Could you check a few things on this model? Use its own coordinates, in mm. A direction names the side the tool comes from. Coordinates: 2 decimals unless noted, no trailing zeros. Write each loop counter-clockwise with the first axis right and the second up, starting at its lowest first coordinate (ties: lowest second). Pieces come first, ordered by that corner, then holes.
```python
from build123d import *

# Parameters (mm, degrees)
CROQUIS1_W                = 5
CROQUIS1_H                = 53
SALIENTE_EXTRUIR1_DEPTH   = 7
SALIENTE_EXTRUIR1_2_DEPTH = 7
CROQUIS3_W                = 53
CROQUIS3_H                = 48
CROQUIS3_W_2              = 33
CROQUIS3_H_2              = 33
CROQUIS3_H_3              = 5
SALIENTE_EXTRUIR2_DEPTH   = 5
CROQUIS4_W                = 53
CROQUIS4_H                = 53
CROQUIS4_W_2              = 43
CROQUIS4_H_2              = 43
SALIENTE_EXTRUIR3_DEPTH   = 32
REDONDEO1_R               = 2
REDONDEO2_R               = 5
CROQUIS5_W                = 5
CROQUIS5_H                = 14
CORTAR_EXTRUIR1_DEPTH     = 32
CROQUIS6_W                = 5
CROQUIS6_H                = 6
CORTAR_EXTRUIR2_DEPTH     = 20
REDONDEO3_R               = 2
CROQUIS7_R                = 4
CROQUIS7_R_2              = 1.75
SALIENTE_EXTRUIR4_DEPTH   = 3
REDONDEO4_R               = 3
REDONDEO7_R               = 3


with BuildPart() as part:
    # Croquis1 → Saliente-Extruir1 (new body)
    with BuildSketch(Plane(origin=(0, 0, 0), x_dir=(0, 1, 0), z_dir=(0, 0, 1))):
        with Locations((-24, 0)):
            Rectangle(CROQUIS1_W, CROQUIS1_H)
    extrude(amount=SALIENTE_EXTRUIR1_DEPTH)



with BuildPart() as body_2:
    # Croquis1 → Saliente-Extruir1 2 (new body)
    with BuildSketch(Plane(origin=(0, 0, 0), x_dir=(0, 1, 0), z_dir=(0, 0, 1))):
        with Locations((24, 0)):
            Rectangle(CROQUIS1_W, CROQUIS1_H)
    extrude(amount=SALIENTE_EXTRUIR1_2_DEPTH)


with BuildPart() as part_1:
    add(part.part)

    add(body_2.part)  # Saliente-Extruir2 merges body 2
    # Croquis3 → Saliente-Extruir2 (add)
    # profile 1 of 2: a face of its own
    with BuildSketch(Plane.XY.offset(7)):
        with Locations((0, 2.5)):
            Rectangle(CROQUIS3_W, CROQUIS3_H)
        Rectangle(CROQUIS3_W_2, CROQUIS3_H_2, mode=Mode.SUBTRACT)
    # profile 2 of 2: a face of its own
    with BuildSketch(Plane.XY.offset(7)):
        with Locations((0, -24)):
            Rectangle(CROQUIS3_W, CROQUIS3_H_3)
    extrude(amount=SALIENTE_EXTRUIR2_DEPTH)

    # Croquis4 → Saliente-Extruir3 (add)
    with BuildSketch(Plane.XY.offset(12)):
        Rectangle(CROQUIS4_W, CROQUIS4_H)
        Rectangle(CROQUIS4_W_2, CROQUIS4_H_2, mode=Mode.SUBTRACT)
    extrude(amount=SALIENTE_EXTRUIR3_DEPTH)

    # Redondeo1
    redondeo1_edges = [part_1.edges().sort_by_distance(p)[0] for p in [
        (21.5, 21.5, 28),
        (-21.5, 21.5, 28),
        (-21.5, -21.5, 28),
        (21.5, -21.5, 28),
    ]]
    fillet(redondeo1_edges, radius=REDONDEO1_R)

    # Redondeo2
    redondeo2_edges = [part_1.edges().sort_by_distance(p)[0] for p in [
        (-26.5, 26.5, 22),
        (26.5, 26.5, 22),
        (26.5, -26.5, 22),
        (-26.5, -26.5, 22),
    ]]
    fillet(redondeo2_edges, radius=REDONDEO2_R - 0.0001)  # a hair under: the kernel refuses the full size

    # Croquis5 → Cortar-Extruir1 (cut)
    with BuildSketch(Plane.XY.offset(44)):
        with Locations((-24, 0)):
            Rectangle(CROQUIS5_W, CROQUIS5_H)
    extrude(amount=-CORTAR_EXTRUIR1_DEPTH, mode=Mode.SUBTRACT)

    # Croquis6 → Cortar-Extruir2 (cut)
    with BuildSketch(Plane.XY.offset(44)):
        with Locations((-24, 10)):
            Rectangle(CROQUIS6_W, CROQUIS6_H)
        with Locations((-24, -10)):
            Rectangle(CROQUIS6_W, CROQUIS6_H)
    extrude(amount=-CORTAR_EXTRUIR2_DEPTH, mode=Mode.SUBTRACT)

    # Redondeo3
    redondeo3_edges = [part_1.edges().sort_by_distance(p)[0] for p in [
        (-24, 7, 12),
        (-24, -7, 12),
        (-24, -13, 24),
        (-24, -7, 24),
        (-24, -13, 44),
        (-24, 13, 44),
        (-24, 7, 24),
        (-24, 13, 24),
        (-26.5, 0, 7),
        (26.5, 0, 7),
    ]]
    fillet(redondeo3_edges, radius=REDONDEO3_R)

    # Croquis7 → Saliente-Extruir4 (add)
    # profile 1 of 2: a face of its own
    with BuildSketch(Plane(origin=(0, 0, 0), x_dir=(0, 1, 0), z_dir=(0, 0, 1))):
        with BuildLine():
            Line((-21.5, 7.5), (-21.5, -7.5))
            Line((-21.5, -7.5), (-9.343708023, -3.829228233))
            ThreePointArc((-9.343708023, -3.829228233), (-14.5, 0), (-9.343708023, 3.829228233))
            Line((-9.343708023, 3.829228233), (-21.5, 7.5))
        make_face()
    # profile 2 of 2: a face of its own
    with BuildSketch(Plane(origin=(0, 0, 0), x_dir=(0, 1, 0), z_dir=(0, 0, 1))):
        with Locations((-10.5, 0)):
            Circle(CROQUIS7_R)
        with Locations(Location((-10.5, 0, 0), (0, 0, 270))):
            Circle(CROQUIS7_R_2, mode=Mode.SUBTRACT)
    saliente_extruir4 = extrude(amount=SALIENTE_EXTRUIR4_DEPTH)

    # Redondeo4
    redondeo4_edges = [part_1.edges().sort_by_distance(p)[0] for p in [
        (7.5, -21.5, 1.5),
        (-7.5, -21.5, 1.5),
    ]]
    fillet(redondeo4_edges, radius=REDONDEO4_R)

    # Simetría5: Saliente-Extruir4 across plane
    add(saliente_extruir4.mirror(Plane.ZX))

    # Redondeo7
    redondeo7_edges = [part_1.edges().sort_by_distance(p)[0] for p in [
        (7.5, 21.5, 1.5),
        (-7.5, 21.5, 1.5),
    ]]
    fillet(redondeo7_edges, radius=REDONDEO7_R)


solid = part_1.part
```
Item 1: If we mould it in two halves opening along Y, with no side actions, what happens to faces 1 (the flat face through (0, -26.5, 22)), 2 (the flat face through (-21.5, -14, 24)), 3 (the flat face through (26.5, 0, 27))? For each: released by +Y, released by -Y, zero draft, split by the parting line, or undercut.
Item 2: I want a section at D-D, the plane z = 28. List the corners of the cut face in (x, y) for me, then the cut area to 3 significant figures.
Item 3: Which directions (+Z, -Z, +X, -X, +Y, -Y) give clear straight access to the entire face, cutting with the end or side of a thin tool? Please do faces 4 (the cylindrical face through (7.961, -20.924, 1.521)), 5 (the flat face through (21.5, 0, 28)), 6 (the cylindrical face through (-23.96, -13.6, 43.43)).
Item 4: I want a section at B-B, the plane y = -2. List the corners of the cut face in (x, z) for me.
Item 5: I want a section at A-A, the plane x = 11.5. List the corners of the cut face in (y, z) for me.
Item 6: If I drill on line 1 along Y through (x, z) = (0, 2); line 2 along X through (y, z) = (19.5, 38), over which ranges is the centre line in solid material (lowest first)?
Item 7: Will these pins go through, and if not, where does the flat tip stop? pin 1 Ø4 at (x, z) = (-24, 34) entering from -Y; pin 2 Ø2.5 at (x, z) = (-25, 20) entering from +Y; pin 3 Ø3 at (x, y) = (16.5, 11) entering from -Z.
Item 8: I want a section at C-C, the plane x = 0. List the corners of the cut face in (y, z) for me, then the cut area to 3 significant figures.
Taken from the geometry:
1. face 1: released by -Y
1. face 2: undercut
1. face 3: zero draft
2. outline: (-26.5, -21.5) arc R5 ccw to (-21.5, -26.5) - (21.5, -26.5) arc R5 ccw to (26.5, -21.5) - (26.5, 21.5) arc R5 ccw to (21.5, 26.5) - (-21.5, 26.5) arc R5 ccw to (-26.5, 21.5) - (-26.5, 13) - (-21.5, 13) - (-21.5, 19.5) arc R2 cw to (-19.5, 21.5) - (19.5, 21.5) arc R2 cw to (21.5, 19.5) - (21.5, -19.5) arc R2 cw to (19.5, -21.5) - (-19.5, -21.5) arc R2 cw to (-21.5, -19.5) - (-21.5, -13) - (-26.5, -13) - close
2. area: 812 mm2
3. face 4: -Z, +X
3. face 5: +Z
3. face 6: +Z, -X
4. outline: (-26.5, 9) arc R2 ccw to (-24.5, 7) - (-16.5, 7) - (-16.5, 12) - (-26.5, 12) - close; (16.5, 7) - (24.5, 7) arc R2 ccw to (26.5, 9) - (26.5, 44) - (21.5, 44) - (21.5, 12) - (16.5, 12) - close
5. outline: (-26.5, 0) - (-21.5, 0) - (-21.5, 7) - (-16.5, 7) - (-16.5, 12) - (-21.5, 12) - (-21.5, 44) - (-26.5, 44) - close; (16.5, 7) - (21.5, 7) - (21.5, 0) - (26.5, 0) - (26.5, 44) - (21.5, 44) - (21.5, 12) - (16.5, 12) - close
6. line 1: y = -26.5 to -12.25, -8.75 to -6.5, 6.5 to 8.75, 12.25 to 26.5
6. line 2: x = -26.5 to -21.5, 21.5 to 26.5
7. pin 1: stops at y = -26.47
7. pin 2: stops at y = 25.97
7. pin 3: stops at z = 7
8. outline: (-26.5, 0) - (-12.25, 0) - (-12.25, 3) - (-21.5, 3) - (-21.5, 7) - (-16.5, 7) - (-16.5, 12) - (-21.5, 12) - (-21.5, 44) - (-26.5, 44) - close; (-8.75, 0) - (-6.5, 0) - (-6.5, 3) - (-8.75, 3) - close; (6.5, 0) - (8.75, 0) - (8.75, 3) - (6.5, 3) - close; (12.25, 0) - (26.5, 0) - (26.5, 44) - (21.5, 44) - (21.5, 12) - (16.5, 12) - (16.5, 7) - (21.5, 7) - (21.5, 3) - (12.25, 3) - close
8. area: 559 mm2
